The listing builds one solid part. Answer for the finished solid, in the listing's coordinates (mm). A direction names the side the tool comes from. Give positions to 0.01 mm unless a question says otherwise; leave off trailing zeros. Loops run counter-clockwise (first coordinate to the right, second up) from the corner with the lowest first, then second, coordinate; pieces in that order, holes last. Notation, with made-up numbers: M 5,38.5 L 11,38.5 A25 ccw 11,74.5 Z; hole C 3,76 d5. An arc over 180 degrees is marked long. Return JSON: item names as keys, results as strings.
from build123d import *

# Parameters (mm, degrees)
F1_DEPTH = 3.6
F2_R     = 0.8
F3_R     = 1.1
F4_R     = 0.3


with BuildPart() as f1:
    # F0 (on Right) → F1 (new body)
    with BuildSketch(Plane.YZ):
        Polygon((-2.066098, 0), (2.066098, 0), (2.066098, 0.3), (-1.805312, 0.3), (-2.351694, 4.187705), (1.463354, 4.054481), (2.066098, 8.963439), (1.768335, 9), (1.199092, 4.363892), (-2.698532, 4.5), align=None)
    extrude(amount=F1_DEPTH)

    # F2
    f2_edges = [f1.edges().sort_by_distance(p)[0] for p in [
        (1.8, -2.351694, 4.187705),
        (1.8, -1.805312, 0.3),
        (1.8, 1.199092, 4.363892),
    ]]
    fillet(f2_edges, radius=F2_R)

    # F3
    f3_edges = [f1.edges().sort_by_distance(p)[0] for p in [
        (1.8, -2.698532, 4.5),
        (1.8, 1.463354, 4.054481),
        (1.8, -2.066098, 0),
    ]]
    fillet(f3_edges, radius=F3_R)

    # F4
    f4_edges = [f1.edges().sort_by_distance(p)[0] for p in [
        (3.6, 1.917216, 8.98172),
        (0, 1.917216, 8.98172),
        (3.6, 2.066098, 0.15),
        (0, 2.066098, 0.15),
    ]]
    fillet(f4_edges, radius=F4_R)


solid = f1.part
(1) Given pin 1 (2 mm diameter, centred on y = -1.5, z = 4.5, fed in from +X), flat-ended and moving along its own axis, determine where the tip first touches the part or whether it passes through.
Values follow:
{"pin 1": "x = 3.6"}
(2) The part is cut by section A-A (y = 0.85). Determine the outline of the cut face in (x, z), and give its area (3 significant figures).
Values follow:
{"outline": "M 0,0 L 3.6,0 L 3.6,0.3 L 0,0.3 Z; M 0,4.15 L 3.6,4.15 L 3.6,4.47 L 0,4.47 Z", "area": "2.25 mm²"}
(3) The part is cut by section B-B (x = 0.95). Determine the outline of the cut face in (y, z).
Values follow:
{"outline": "M -2.52,3.2 L -2.2,0.95 A1.1 ccw -1.11,0 L 2.07,0 L 2.07,0.3 L -1.11,0.3 A0.8 cw -1.9,0.99 L -2.22,3.24 A0.8 cw -1.4,4.15 L 0.46,4.09 A1.1 ccw 1.59,5.05 L 2.07,8.96 L 1.77,9 L 1.29,5.09 A0.8 cw 0.47,4.39 L -1.39,4.45 A1.1 ccw Z"}
(4) The part is cut by section D-D (y = -1.75). Determine the outline of the cut face in (x, z), and give its area (3 significant figures).
Values follow:
{"outline": "M 0,0.21 L 3.6,0.21 L 3.6,0.62 L 0,0.62 Z; M 0,4.09 L 3.6,4.09 L 3.6,4.41 L 0,4.41 Z", "area": "2.64 mm²"}
(5) Straight lines are drawn through the part: line 1 along Z through (x, y) = (1.25, -0.9); line 2 along Z through (x, y) = (2.5, 1); line 3 along Y through (x, z) = (2.8, 1.75). For each, find the intervals that lie inside material, in ascending order.
Values follow:
{"line 1": "0 to 0.3, 4.14 to 4.44", "line 2": "0 to 0.3, 4.21 to 4.57", "line 3": "-2.31 to -2.01"}
(6) Determine the mould class of faces 1 (the flat face through (1.77, -2.06, 2.1)), 2 (the flat face through (2, 0, 0)), 3 (the cylindrical face through (1.825, 1.02, 4.586)) for opening direction Z: released by +Z, released by -Z, zero draft, split by the parting line, or undercut.
Values follow:
{"face 1": "undercut", "face 2": "released by -Z", "face 3": "released by +Z"}
(7) A tool of negligible diameter and unlimited length cuts with its end or side. For faces 4 (the flat face through (1.775, 1.823, 6.982)), 5 (the flat face through (1.77, -2.36, 2.09)), 6 (the cylindrical face through (1.83, -2.03, 3.88)), from which of +Z, -Z, +X, -X, +Y, -Y can it reach the whole face along a straight path? Write none if from no direction.
Values follow:
{"face 4": "+X, -X, +Y", "face 5": "-Z, +X, -X, -Y", "face 6": "+X, -X"}
(8) The part is cut by section C-C (z = 7.5). Determine the outline of the cut face in (x, y), and give its area (3 significant figures).
Values follow:
{"outline": "M 0,1.58 L 3.6,1.58 L 3.6,1.89 L 0,1.89 Z", "area": "1.09 mm²"}
